Autodesk Inventor part; units mm, degrees
ref_plane "ROD_BA_XY" through (10, 0, 0) normal (-1, 0, 0) x (0, 0, -1)
ref_plane "ROD_BA_YZ" through (10, 0, 0) normal (0, 0, -1) x (0, -1, 0)
ref_plane "ROD_BA_ZX" through (10, 0, 0) normal (0, -1, 0) x (-1, 0, 0)
sketch "Sketch_5" plane through (0, 0, 0) normal (0, 0, 1) x (1, 0, 0)
  line L0 (245.5, 0) -> (0, 0)
  line L1 (0, 0) -> (0, 2.0095)
  line L2 (0, 2.0095) -> (0.4905, 2.5)
  line L3 (0.4905, 2.5) -> (15, 2.5)
  line L4 (15, 2.5) -> (15, 2.067)
  line L5 (15, 2.067) -> (16.5, 2.067)
  line L6 (16.5, 2.067) -> (16.5, 2.5)
  line L7 (16.5, 2.5) -> (240.5, 2.5)
  line L8 (240.5, 2.5) -> (240.5, 8)
  line L9 (240.5, 8) -> (245.5, 8)
  line L10 (245.5, 8) -> (245.5, 0)
  line L11 (245.5, 0) -> (0, 0)
revolve "Revolution1" add sketch "Sketch_5" angle 360 about axis through (245.5, 0, 0) along (1, 0, 0)
thread "Thread1"
ref_plane "ROD_BA_XY" through (10, 0, 0) normal (-1, 0, 0) x (0, 0, -1)
ref_plane "ROD_BA_YZ" through (10, 0, 0) normal (0, 0, -1) x (0, -1, 0)
ref_plane "ROD_BA_ZX" through (10, 0, 0) normal (0, -1, 0) x (-1, 0, 0)
ref_plane "ROD_BODY_XY" through (28, 0, 0) normal (-1, 0, 0) x (0, 0, -1)
ref_plane "ROD_BODY_YZ" through (28, 0, 0) normal (0, 0, -1) x (0, -1, 0)
ref_plane "ROD_BODY_ZX" through (28, 0, 0) normal (0, -1, 0) x (-1, 0, 0)
ref_plane "rodnt1_XY" through (7.5, 0, 0) normal (1, 0, 0) x (0, 0, -1)
ref_plane "rodnt1_YZ" through (7.5, 0, 0) normal (0, 0, -1) x (0, 1, 0)
ref_plane "rodnt1_ZX" through (7.5, 0, 0) normal (0, 1, 0) x (1, 0, 0)
properties part number "CJ2B16-200Z_ROD" material "鉄、鋳鉄"
Input: part model. Units: mm. Frame: model coordinates. A direction names the side the tool comes from. Coordinates: 2 decimals unless noted, no trailing zeros. Write each loop counter-clockwise with the first axis right and the second up, starting at its lowest first coordinate (ties: lowest second). Pieces come first, ordered by that corner, then holes.
1) Mould query, pull axis X, two halves, no side actions, for faces 4 (the cylindrical face through (7.85, -0.54, -2.44)), 5 (the flat face through (240.5, -2, -2)), 6 (the flat face through (15, -1, 2)). Classes: pulls with the +X half, pulls with the -X half, needs draft (parallel to the pull), parting line crosses it, or undercut.
2) Material intervals for line 1 along X through (y, z) = (-5, -2); line 2 along Y through (x, z) = (227, 0.25); line 3 along Y through (x, z) = (194, -1.5), sorted ascending.
3) Section A-A on z = 0. Output: boundary loops of the cut face in (x, y), and give its area (3 significant figures).
4) Section C-C on x = 221.5. Output: boundary loops of the cut face in (y, z), and give its area (3 significant figures).
5) Pin query (flat end, axial travel): pin 1 Ø1.5 at (x, z) = (51, 0) entering from +Y; pin 2 Ø2 at (y, z) = (-3, 2) entering from -X; pin 3 Ø5 at (x, y) = (74.5, 4.5) entering from +Z. Return the tip coordinate at first contact, or that it passes through.
6) Set-up query: faces 1 (the cylindrical face through (130.07, -0.54, -2.44)), 2 (the cylindrical face through (15.76, -1.64, -1.26)), 3 (the flat face through (0, 0, 0)). Return all of +Z, -Z, +X, -X, +Y, -Y with unobstructed straight access to the full face (end or side cutting, diameter ignored); none if empty.
Check result:
1. face 4: needs draft
1. face 5: pulls with the -X half
1. face 6: undercut
2. line 1: x = 240.5 to 245.5
2. line 2: y = -2.49 to 2.49
2. line 3: y = -2 to 2
3. outline: (0, -2.01) - (0.49, -2.5) - (15, -2.5) - (15, -2.07) - (16.5, -2.07) - (16.5, -2.5) - (240.5, -2.5) - (240.5, -8) - (245.5, -8) - (245.5, 8) - (240.5, 8) - (240.5, 2.5) - (16.5, 2.5) - (16.5, 2.07) - (15, 2.07) - (15, 2.5) - (0.49, 2.5) - (0, 2.01) - close
3. area: 1,280 mm2
4. outline: circle Ø5 at (0, 0)
4. area: 19.6 mm2
5. pin 1: stops at y = 2.5
5. pin 2: stops at x = 240.5
5. pin 3: stops at z = 1.5
6. face 1: -X
6. face 2: none
6. face 3: +Z, -Z, -X, +Y, -Y
